```python
from build123d import *

# Parameters (mm, degrees)
EXTRUDE_1_DEPTH     = 7
SKETCH_2_R          = 1.15
CUT_EXTRUDE_1_DEPTH = 10
SKETCH_5_R          = 1.15
CUT_EXTRUDE_3_DEPTH = 10
FILLET_1_R          = 1.1
CUT_EXTRUDE_4_DEPTH = 1


with BuildPart() as part:
    # Эскиз1 → Бобышка-Вытянуть1 (new body)
    with BuildSketch(Plane.ZY.offset(-220)):
        Polygon((-2.700000149, 10), (-2.700000149, 5.5), (2.700000149, 5.5), (2.700000149, 10), (10.000000149, 10), (10.000000149, 2.700000104), (5.500000149, 2.700000104), (5.500000149, -2.700000194), (10.000000149, -2.700000194), (10.000000149, -10), (40.000000149, -10), (40.000000149, -5), (20.000000149, 15), (-8.500000149, 15), (-8.500000149, 10), align=None)
    extrude(amount=EXTRUDE_1_DEPTH)

    # Эскиз2 → Вырез-Вытянуть1 (cut)
    with BuildSketch(Plane(origin=(0, 17.500000075, 17.500000075), x_dir=(1, 0, 0), z_dir=(0, 0.7071067811865489, 0.7071067811865462))):
        with Locations(Location((216.5, -14.177669635, 0), (0, 0, 270))):
            Circle(SKETCH_2_R)
    extrude(amount=-CUT_EXTRUDE_1_DEPTH, mode=Mode.SUBTRACT)

    # Эскиз5 → Вырез-Вытянуть3 (cut)
    with BuildSketch(Plane(origin=(0, 17.500000075, 17.500000075), x_dir=(1, 0, 0), z_dir=(0, 0.7071067811865489, 0.7071067811865462))):
        with Locations(Location((216.5, -8.856601823, 0), (0, 0, 270))):
            Circle(SKETCH_5_R)
        with Locations(Location((216.5, -19.498737447, 0), (0, 0, 270))):
            Circle(SKETCH_5_R)
    extrude(amount=-CUT_EXTRUDE_3_DEPTH, mode=Mode.SUBTRACT)

    # Скругление1
    fillet_1_edges = [part.edges().sort_by_distance(p)[0] for p in [
        (220, 12.5, -8.500000149),
        (220, 15, 5.75),
        (220, 5, 30.000000149),
        (220, -7.5, 40.000000149),
        (220, -10, 25.000000149),
        (216.5, 15, -8.500000149),
        (216.5, 15, 20.000000149),
        (216.5, -5, 40.000000149),
        (216.5, -10, 40.000000149),
        (213, -10, 25.000000149),
        (216.5, 8.288046533, 26.711953616),
        (213, -7.5, 40.000000149),
        (216.5, 4.5254834, 30.474516749),
        (216.5, 12.050609665, 22.949390484),
        (213, 5, 30.000000149),
        (213, 15, 5.75),
        (213, 12.5, -8.500000149),
    ]]
    fillet(fillet_1_edges, radius=FILLET_1_R)

    # Эскиз6 → Вырез-Вытянуть4 (cut)
    with BuildSketch(Plane(origin=(0, 17.500000075, 17.500000075), x_dir=(1, 0, 0), z_dir=(0, 0.707106781186549, 0.7071067811865462))):
        with BuildLine():
            add(Edge.make_bspline(
                [(216.502435065, -25.86417034), (216.536563033, -25.865221496), (216.60371255, -25.867289731), (216.702509896, -25.880193482), (216.797502694, -25.90299359), (216.888288666, -25.935893054), (216.976029709, -25.976281211), (217.058990215, -26.027141192), (217.138113432, -26.086933249), (217.212888867, -26.154484411), (217.281279441, -26.228230082), (217.341260408, -26.307127858), (217.392409957, -26.389601594), (217.434342901, -26.476295263), (217.465809589, -26.566855017), (217.488759341, -26.661138444), (217.502763598, -26.759314764), (217.50470136, -26.826246251), (217.505681818, -26.860111899)],
                knots=[0, 0, 0, 0, 1.041766559, 2.049759373, 3.035273881, 4.017460812, 4.992853655, 5.978644954, 6.981244037, 8.016212218, 9.050653059, 10.046665791, 11.0367719, 12.008241014, 12.979885633, 13.957373994, 14.966482649, 16, 16, 16, 16], degree=3))
            add(Edge.make_bspline(
                [(217.505681818, -26.860111899), (217.503432714, -26.907658615), (217.498865545, -27.004209893), (217.462636232, -27.14864688), (217.404638062, -27.293498456), (217.350815973, -27.385635252), (217.323051948, -27.433163847)],
                knots=[0, 0, 0, 0, 0.935810177, 1.900313523, 2.916880626, 4, 4, 4, 4], degree=3))
            Line((217.323051948, -27.433163847), (216.058441558, -29.448585925))
            Line((216.058441558, -29.448585925), (217.305194805, -29.448585925))
            add(Edge.make_bspline(
                [(217.305194805, -29.448585925), (217.320952575, -29.449106667), (217.350647274, -29.450087979), (217.392201576, -29.460065459), (217.427876696, -29.475843079), (217.456618488, -29.499740234), (217.478865792, -29.529855517), (217.495475433, -29.566218207), (217.503813047, -29.609475843), (217.505033813, -29.640114546), (217.505681818, -29.656378132)],
                knots=[0, 0, 0, 0, 1.14095523, 2.150070966, 3.080760824, 3.945153579, 4.828279774, 5.776800167, 6.819884637, 8, 8, 8, 8], degree=3))
            add(Edge.make_bspline(
                [(217.505681818, -29.656378132), (217.505033813, -29.672641719), (217.503813047, -29.703280421), (217.495475433, -29.746538058), (217.478865792, -29.782900748), (217.456618488, -29.813016031), (217.427876696, -29.836913185), (217.392201576, -29.852690806), (217.350647274, -29.862668286), (217.320952575, -29.863649598), (217.305194805, -29.86417034)],
                knots=[0, 0, 0, 0, 1.180115363, 2.223199833, 3.171720226, 4.054846421, 4.919239176, 5.849929034, 6.85904477, 8, 8, 8, 8], degree=3))
            Line((217.305194805, -29.86417034), (215.699675325, -29.86417034))
            add(Edge.make_bspline(
                [(215.699675325, -29.86417034), (215.683933164, -29.863567282), (215.65432857, -29.862433176), (215.61274605, -29.853541174), (215.577095512, -29.83854485), (215.548270828, -29.815522562), (215.52624531, -29.786349963), (215.509347256, -29.751498386), (215.501114388, -29.71004685), (215.499853401, -29.680755827), (215.499188312, -29.665306704)],
                knots=[0, 0, 0, 0, 1.166197201, 2.193142131, 3.13613798, 4.007040048, 4.893738447, 5.826868706, 6.853813636, 8, 8, 8, 8], degree=3))
            add(Edge.make_bspline(
                [(215.499188312, -29.665306704), (215.500545826, -29.64516914), (215.503297006, -29.604357748), (215.522659217, -29.568308455), (215.532467532, -29.550046964)],
                knots=[0, 0, 0, 0, 0.986859896, 2, 2, 2, 2], degree=3))
            Line((215.532467532, -29.550046964), (217.004058442, -27.205891119))
            add(Edge.make_bspline(
                [(217.004058442, -27.205891119), (217.019421898, -27.179479546), (217.049535538, -27.127710686), (217.081108754, -27.045100631), (217.100727999, -26.961408789), (217.103386527, -26.905128284), (217.104707792, -26.877157353)],
                knots=[0, 0, 0, 0, 1.051688452, 2.061396058, 3.036530382, 4, 4, 4, 4], degree=3))
            add(Edge.make_bspline(
                [(217.104707792, -26.877157353), (217.104401122, -26.85682656), (217.103796871, -26.816767517), (217.094194077, -26.758125541), (217.080278553, -26.701710753), (217.06225054, -26.647064491), (217.036248612, -26.595477549), (217.005447031, -26.546108342), (216.969585749, -26.498575919), (216.928166943, -26.454376736), (216.883491772, -26.413514712), (216.836140094, -26.377343683), (216.786377846, -26.347059109), (216.733958309, -26.322779543), (216.679476241, -26.302981965), (216.622306603, -26.289304254), (216.563021254, -26.280952172), (216.52275483, -26.280156353), (216.502435065, -26.279754756)],
                knots=[0, 0, 0, 0, 1.033348237, 2.036071235, 3.014398079, 3.989620349, 4.956253624, 5.945657129, 6.947907479, 7.980521803, 9.023273023, 10.025523372, 11.007717137, 11.980799265, 12.960577993, 13.952277545, 14.966651763, 16, 16, 16, 16], degree=3))
            add(Edge.make_bspline(
                [(216.502435065, -26.279754756), (216.474131666, -26.281380338), (216.417101513, -26.284655817), (216.333088605, -26.309743664), (216.250805948, -26.34927274), (216.170745637, -26.405681834), (216.092865656, -26.478006076), (216.016660073, -26.565648709), (215.941528023, -26.668471995), (215.896266541, -26.744704834), (215.872564935, -26.784624886)],
                knots=[0, 0, 0, 0, 0.802989863, 1.617990652, 2.470504536, 3.387253077, 4.388154308, 5.482780424, 6.681833993, 8, 8, 8, 8], degree=3))
            add(Edge.make_bspline(
                [(215.872564935, -26.784624886), (215.86306896, -26.799363595), (215.844430415, -26.828292495), (215.803113907, -26.859883264), (215.753633036, -26.878477726), (215.718243076, -26.880805952), (215.699675325, -26.882027483)],
                knots=[0, 0, 0, 0, 1.002746525, 1.968174689, 2.933979409, 4, 4, 4, 4], degree=3))
            add(Edge.make_bspline(
                [(215.699675325, -26.882027483), (215.683944176, -26.881398221), (215.65436029, -26.880214837), (215.612530112, -26.871627302), (215.577243985, -26.855463651), (215.54856423, -26.832651565), (215.525752144, -26.803971809), (215.509588493, -26.768685682), (215.501000958, -26.726855504), (215.499817573, -26.697271619), (215.499188312, -26.68154047)],
                knots=[0, 0, 0, 0, 1.161746488, 2.184772153, 3.132421671, 4, 4.867578329, 5.815227847, 6.838253512, 8, 8, 8, 8], degree=3))
            add(Edge.make_bspline(
                [(215.499188312, -26.68154047), (215.500057235, -26.667034119), (215.501750412, -26.638767178), (215.512037575, -26.612397121), (215.517045455, -26.599559951)],
                knots=[0, 0, 0, 0, 1.026382828, 2, 2, 2, 2], degree=3))
            add(Edge.make_bspline(
                [(215.517045455, -26.599559951), (215.532691663, -26.569619946), (215.563235107, -26.511173146), (215.613503334, -26.42818001), (215.663857233, -26.349944946), (215.718169501, -26.27854673), (215.772733268, -26.211839023), (215.829908634, -26.151577787), (215.888717549, -26.096804028), (215.949127, -26.047243019), (216.012040101, -26.004133199), (216.076479009, -25.966441952), (216.142887069, -25.934603446), (216.211632658, -25.909733515), (216.281472428, -25.889165211), (216.353357859, -25.874254529), (216.427316836, -25.866457749), (216.477256972, -25.864937033), (216.502435065, -25.86417034)],
                knots=[0, 0, 0, 0, 1.247331567, 2.434954234, 3.582379257, 4.681579802, 5.746075506, 6.763961717, 7.746761029, 8.712805542, 9.646898869, 10.560400761, 11.467760656, 12.362486931, 13.257436386, 14.155004042, 15.069816711, 16, 16, 16, 16], degree=3))
        make_face()
    extrude(amount=-CUT_EXTRUDE_4_DEPTH, mode=Mode.SUBTRACT)


solid = part.part
```
Check sheet for the modelled part. Datum: model origin and axes. Units: mm. A direction names the side the tool comes from. Give positions to 0.01 mm unless a question says otherwise; leave off trailing zeros. Write each loop counter-clockwise with the first axis right and the second up, starting at its lowest first coordinate (ties: lowest second). Pieces come first, ordered by that corner, then holes.
Item 1: Scan lines: L1, parallel to Y at x = 215.5, z = 7.5; L2, parallel to Z at x = 216, y = 7; L3, parallel to Z at x = 219.25, y = 9.25. Record each from-to range of solid material in increasing order.
Item 2: Cross-section at A-A (z = 4). Enter the section's corners in (x, y).
Item 3: Cross-section at C-C (y = -6.5). Enter the section's corners in (x, z), and give its area (3 significant figures).
Item 4: Access from +Z, -Z, +X, -X, +Y, -Y to the whole of each face (thin tool, end or side, straight path). Record for faces 5 (the face through (216.52, 0.42, 20.44)), 6 (the face through (217, 0, 5.5)), 7 (the face through (217, 6, 10)), 8 (the face through (213.314, 14.669, 5.884)).
Item 5: Gauge pin test, flat ends, axial feed: pin 1 (3.5 mm diameter, centred on x = 218, y = 8, fed in from -Z); pin 2 (2.5 mm diameter, centred on x = 216, y = -0.5, fed in from -Z); pin 3 (2.5 mm diameter, centred on x = 217, z = -1, fed in from -Y). Record the tip position at first contact, or that the pin passes through.
Item 6: Draft check along Z on faces 1 (the face through (217, 2.7, 8)), 2 (the face through (213.314, -7.154, 39.669)), 3 (the face through (217, 8, -2.7)), 4 (the face through (217, 10, 6)). Enter one of: released by +Z, released by -Z, zero draft, split by the parting line, or undercut.
Item 7: Cross-section at B-B (y = 6.5). Count the separate pieces of the cut face and the enclosed holes in it, and give its area (3 significant figures).
Report:
1. L1: y = -2.7 to 2.7, 10 to 15
1. L2: z = -2.7 to 2.7, 10 to 18.06, 20.99 to 25.59
1. L3: z = -2.7 to 2.7, 10 to 25.67
2. outline: (213, 10) - (220, 10) - (220, 13.9) arc R1.1 ccw to (218.9, 15) - (214.1, 15) arc R1.1 ccw to (213, 13.9) - close
3. outline: (213, 10) - (220, 10) - (220, 38.9) arc R1.1 ccw to (218.9, 40) - (214.1, 40) arc R1.1 ccw to (213, 38.9) - close
3. area: 209 mm2
4. face 5: none
4. face 6: -Z, +X, -X, -Y
4. face 7: +X, -X
4. face 8: +Z, -Z, -X, +Y
5. pin 1: stops at z = -2.7
5. pin 2: stops at z = 5.5
5. pin 3: stops at y = 5.5
6. face 1: zero draft
6. face 2: released by +Z
6. face 3: released by -Z
6. face 4: undercut
7. separate pieces: 2
7. enclosed holes: 1
7. area: 153 mm2
